```python
from build123d import *

# Parameters (mm, degrees)
F0_R      = 110
F0_R_2    = 1.25
F0_R_3    = 11
F0_R_4    = 1.5875
F1_DEPTH  = 1
F2_R      = 110
F2_W      = 150
F2_H      = 90
F3_DEPTH  = 1.001
F4_R      = 1.5875
F5_DEPTH  = 1.001
F6_W      = 21
F6_H      = 90
F7_DEPTH  = 1.001
F8_W      = 149
F8_H      = 110
F8_W_2    = 129
F8_H_2    = 90
F9_DEPTH  = 1
F11_DEPTH = 25


with BuildPart() as f1:
    # F0 (on Top) → F1 (new body)
    with BuildSketch(Plane.XY):
        Circle(F0_R)
        with Locations((-11.5, -11.5)):
            Circle(F0_R_2, mode=Mode.SUBTRACT)
        with Locations((11.5, -11.5)):
            Circle(F0_R_2, mode=Mode.SUBTRACT)
        with Locations((-11.5, 11.5)):
            Circle(F0_R_2, mode=Mode.SUBTRACT)
        Circle(F0_R_3, mode=Mode.SUBTRACT)
        with Locations((11.5, 11.5)):
            Circle(F0_R_2, mode=Mode.SUBTRACT)
        with Locations((50, 0)):
            Circle(F0_R_4, mode=Mode.SUBTRACT)
    extrude(amount=F1_DEPTH)

    # F2 (on Top) → F3 (cut, through all)
    with BuildSketch(Plane.XY):
        Circle(F2_R)
        Rectangle(F2_W, F2_H, mode=Mode.SUBTRACT)
    extrude(amount=F3_DEPTH, mode=Mode.SUBTRACT)

    # F4 (on Top) → F5 (cut, through all)
    with BuildSketch(Plane.XY):
        with Locations((-50, 41)):
            Circle(F4_R)
        with Locations((-50, -41)):
            Circle(F4_R)
        with Locations((71, -41)):
            Circle(F4_R)
        with Locations((71, 41)):
            Circle(F4_R)
    extrude(amount=F5_DEPTH, mode=Mode.SUBTRACT)

    # F6 (on Top) → F7 (cut, through all)
    with BuildSketch(Plane.XY):
        with Locations((-64.5, 0)):
            Rectangle(F6_W, F6_H)
    extrude(amount=F7_DEPTH, mode=Mode.SUBTRACT)

    # F8 (on Top) → F9 (join, through all)
    with BuildSketch(Plane.XY):
        with Locations((10.5, 0)):
            Rectangle(F8_W, F8_H)
        with Locations((10.5, 0)):
            Rectangle(F8_W_2, F8_H_2, mode=Mode.SUBTRACT)
    extrude(amount=F9_DEPTH)

    # F10 (on Top) → F11 (cut)
    with BuildSketch(Plane.XY):
        with BuildLine():
            Line((65, 55), (-44, 55))
            ThreePointArc((-44, 55), (10.5, 25), (65, 55))
        make_face()
        with BuildLine():
            ThreePointArc((-64, -35), (-24, 0), (-64, 35))
            Line((-64, 35), (-64, -35))
        make_face()
        with BuildLine():
            ThreePointArc((65, -55), (10.5, -25), (-44, -55))
            Line((-44, -55), (65, -55))
        make_face()
        with BuildLine():
            Line((85, -35), (85, 35))
            ThreePointArc((85, 35), (60, 0), (85, -35))
        make_face()
    extrude(amount=F11_DEPTH, mode=Mode.SUBTRACT)


solid = f1.part
```
For this review, take the finished solid that the model builds, in its own axes (mm). Coordinates: 2 decimals unless noted, no trailing zeros. Order: outer loops, then holes, each group sorted by start corner. A loop starts at its lowest first (then second) coordinate and runs counter-clockwise, first axis right, second up. Notation, with made-up numbers: (-37.75, 9) -> (-30.75, 9) arc R25 ccw to (-30.75, 33) -> close; hole circle Ø6 at (75, 82). An arc over 180 degrees is marked (long way). Use CSV: the item, a comma, the result in double quotes. Start each with the question number.
Item 1: Wall thickness on probe 1 along Y at (x, z) = (11.5, 0.5); probe 2 along X at (y, z) = (-0.5, 0.4); probe 3 along Y at (x, z) = (71, 0.35): over which ranges is each line inside the solid? List them lowest first.
Item 2: Draft analysis for pull direction X (two halves, no side actions). For faces 1 (the face through (51.514, 0.477, 0.493)), 2 (the face through (11.409, -25.006, 0.493)), 3 (the face through (60.006, 0.643, 0.493)), 4 (the face through (26, 1, 1)), state which applies: pulls with the +X half, pulls with the -X half, needs draft (parallel to the pull), parting line crosses it, or undercut.
Item 3: We need section D-D, the plane y = -37. Give the boundary of the cut face in (x, z).
Item 4: We need section C-C, the plane x = 50. Give the boundary of the cut face in (y, z), then the cut area to 3 significant figures.
Item 5: We need section A-A, the plane z = 0.3. Give the number of separate pieces and of enclosed holes in the cut face, then the cut area to 3 significant figures.
Item 6: We need section B-B, the plane y = 0. Give the boundary of the cut face in (x, z).
Derived:
1,probe 1,"y = -25.01 to -12.75, -10.25 to 10.25, 12.75 to 25.01"
1,probe 2,"x = -24 to -10.99, 10.99 to 48.49, 51.51 to 60"
1,probe 3,"y = -55 to -42.59, -39.41 to -26.32, 26.32 to 39.41, 42.59 to 55"
2,face 1,"undercut"
2,face 2,"undercut"
2,face 3,"pulls with the +X half"
2,face 4,"needs draft"
3,outline,"(-64, 0) -> (-26.97, 0) -> (-26.97, 1) -> (-64, 1) -> close; (47.97, 0) -> (85, 0) -> (85, 1) -> (47.97, 1) -> close"
4,outline,"(-38.51, 0) -> (-1.59, 0) -> (-1.59, 1) -> (-38.51, 1) -> close; (1.59, 0) -> (38.51, 0) -> (38.51, 1) -> (1.59, 1) -> close"
4,area,"73.8 mm^2"
5,separate pieces,"1"
5,enclosed holes,"10"
5,area,"7,770 mm^2"
6,outline,"(-24, 0) -> (-11, 0) -> (-11, 1) -> (-24, 1) -> close; (11, 0) -> (48.41, 0) -> (48.41, 1) -> (11, 1) -> close; (51.59, 0) -> (60, 0) -> (60, 1) -> (51.59, 1) -> close"
